```python
from build123d import *

# Parameters (mm, degrees)
BOSS_EXTRUDE2_DEPTH      = 0.9
BOSS_EXTRUDE2_DEPTH_BACK = 0.9
SKETCH1_R                = 2.5
SKETCH1_R_2              = 1.6


with BuildPart() as part:
    # Sketch1 → Boss-Extrude2 (new, two sides: drawn at the far end of the back side and taken through both)
    # profile 1 of 3: a face of its own
    with BuildSketch(Plane.XY.offset(-BOSS_EXTRUDE2_DEPTH_BACK)):
        with BuildLine():
            Line((7.5, 3.5), (-7.5, 3.5))
            ThreePointArc((-7.5, 3.5), (-5.732233047, 2.767766953), (-5, 1))
            ThreePointArc((-5, 1), (-5.732233047, -0.767766953), (-7.5, -1.5))
            Line((-7.5, -1.5), (7.5, -1.5))
            ThreePointArc((7.5, -1.5), (5, 1), (7.5, 3.5))
        make_face()
    # profile 2 of 3: a face of its own
    with BuildSketch(Plane.XY.offset(-BOSS_EXTRUDE2_DEPTH_BACK)):
        with Locations((-7.5, 1)):
            Circle(SKETCH1_R)
        with Locations((-7.5, 1)):
            Circle(SKETCH1_R_2, mode=Mode.SUBTRACT)
    # profile 3 of 3: a face of its own
    with BuildSketch(Plane.XY.offset(-BOSS_EXTRUDE2_DEPTH_BACK)):
        with Locations((7.5, 1)):
            Circle(SKETCH1_R)
        with Locations((7.5, 1)):
            Circle(SKETCH1_R_2, mode=Mode.SUBTRACT)
    extrude(amount=BOSS_EXTRUDE2_DEPTH + BOSS_EXTRUDE2_DEPTH_BACK)


solid = part.part
```
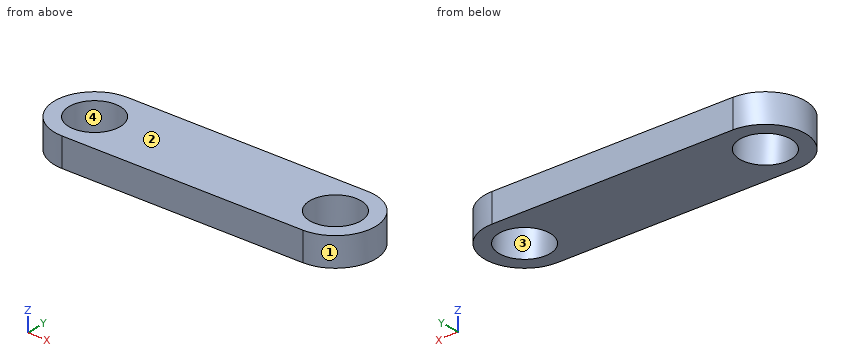
Build history of the part. All positions in model axes, mm. Face numbers are marked on the shaded views. Round coordinates to 2 decimals unless told otherwise and drop trailing zeros. Order: outer loops, then holes, each group sorted by start corner. A loop starts at its lowest first (then second) coordinate and runs counter-clockwise, first axis right, second up. Notation, with made-up numbers: (-7.5, -33) - (11.5, -33) arc R27 cw to (11.5, -17) - close; hole circle Ø9 at (37, 66.25). An arc over 180 degrees is marked (long way). Use a Markdown table: item, result.
1) Saw through at C-C on y = 0.8. Write the cut outline in (x, z), and give its area (3 significant figures).
Recorded:
| item | result |
|---|---|
| outline | (-9.99, -0.9) - (-9.09, -0.9) - (-9.09, 0.9) - (-9.99, 0.9) - close; (-5.91, -0.9) - (5.91, -0.9) - (5.91, 0.9) - (-5.91, 0.9) - close; (9.09, -0.9) - (9.99, -0.9) - (9.99, 0.9) - (9.09, 0.9) - close |
| area | 24.5 mm² |
2) Saw through at B-B on z = 0.3. Write the cut outline in (x, y).
Recorded:
| item | result |
|---|---|
| outline | (-7.5, -1.5) - (7.5, -1.5) arc R2.5 ccw to (7.5, 3.5) - (-7.5, 3.5) arc R2.5 ccw to start; hole circle Ø3.2 at (-7.5, 1); hole circle Ø3.2 at (7.5, 1) |
3) Pull direction X, two halves, no side cores. Call the marked faces 1, 2, 3 and 4: pulls with the +X half, pulls with the -X half, needs draft (parallel to the pull), parting line crosses it, or undercut.
Recorded:
| item | result |
|---|---|
| face 1 | pulls with the +X half |
| face 2 | needs draft |
| face 3 | undercut |
| face 4 | undercut |
4) Saw through at D-D on x = -7.75. Write the cut outline in (y, z), and give its area (3 significant figures).
Recorded:
| item | result |
|---|---|
| outline | (-1.49, -0.9) - (-0.58, -0.9) - (-0.58, 0.9) - (-1.49, 0.9) - close; (2.58, -0.9) - (3.49, -0.9) - (3.49, 0.9) - (2.58, 0.9) - close |
| area | 3.27 mm² |
5) Saw through at A-A on x = 6.5. Write the cut outline in (y, z), and give its area (3 significant figures).
Recorded:
| item | result |
|---|---|
| outline | (-1.5, -0.9) - (-0.25, -0.9) - (-0.25, 0.9) - (-1.5, 0.9) - close; (2.25, -0.9) - (3.5, -0.9) - (3.5, 0.9) - (2.25, 0.9) - close |
| area | 4.50 mm² |
6) Wall check: L1, parallel to X at y = 0.95, z = -0.35; L2, parallel to Y at x = -7.5, z = 0.5; L3, parallel to X at y = -0.9, z = -0.4. Give the ranges that are in metal, low to high.
Recorded:
| item | result |
|---|---|
| L1 | x = -10 to -9.1, -5.9 to 5.9, 9.1 to 10 |
| L2 | y = -1.5 to -0.6, 2.6 to 3.5 |
| L3 | x = -9.12 to 9.12 |
7) Flat gauge pin, fed straight in: pin 1 Ø1.9 at (x, y) = (7.5, 1) entering from +Z. Where does the tip first touch, or does it go through?
Recorded:
| item | result |
|---|---|
| pin 1 | passes through |
